Work out the finished part from the listing and answer in its coordinate system (mm). Round coordinates to 2 decimals unless told otherwise and drop trailing zeros. Write each loop counter-clockwise with the first axis right and the second up, starting at its lowest first coordinate (ties: lowest second). Pieces come first, ordered by that corner, then holes. Notation, with made-up numbers: (76, 21) - (135, 21) arc R27 cw to (135, 48) - close; hole circle Ø2 at (-19.75, 52.5). An arc over 180 degrees is marked (long way). Answer as a JSON object with one key per item and string values.
```python
from build123d import *

# Parameters (mm, degrees)
SKETCH2_W           = 200
SKETCH2_H           = 20
BOSS_EXTRUDE1_DEPTH = 3
SKETCH3_R           = 3
CUT_EXTRUDE1_DEPTH  = 202.019899512
SKETCH4_R           = 3
CUT_EXTRUDE2_DEPTH  = 202.019899512
FILLET1_R           = 10
FILLET2_R           = 10
SKETCH6_R           = 3
CUT_EXTRUDE3_DEPTH  = 202.019899512


with BuildPart() as part:
    # Sketch2 → Boss-Extrude1 (new body)
    with BuildSketch(Plane(origin=(0, 0, 0), x_dir=(1, 0, 0), z_dir=(0, 1, 0))):
        with Locations((100, 10)):
            Rectangle(SKETCH2_W, SKETCH2_H)
    extrude(amount=BOSS_EXTRUDE1_DEPTH)

    # Sketch3 → Cut-Extrude1 (cut, through all)
    with BuildSketch(Plane(origin=(0, 3, 0), x_dir=(1, 0, 0), z_dir=(0, 1, 0))):
        with Locations(Location((9, 10, 0), (0, 0, 270))):
            Circle(SKETCH3_R)
    extrude(amount=-CUT_EXTRUDE1_DEPTH, mode=Mode.SUBTRACT)

    # Sketch4 → Cut-Extrude2 (cut, through all)
    with BuildSketch(Plane(origin=(0, 3, 0), x_dir=(1, 0, 0), z_dir=(0, 1, 0))):
        with Locations(Location((191, 10, 0), (0, 0, 270))):
            Circle(SKETCH4_R)
    extrude(amount=-CUT_EXTRUDE2_DEPTH, mode=Mode.SUBTRACT)

    # Fillet1
    fillet1_edges = [part.edges().sort_by_distance(p)[0] for p in [
        (0, 1.5, -20),
        (0, 1.5, 0),
    ]]
    fillet(fillet1_edges, radius=FILLET1_R - 0.0001)  # a hair under: the kernel refuses the full size

    # Fillet2
    fillet2_edges = [part.edges().sort_by_distance(p)[0] for p in [
        (200, 1.5, -20),
        (200, 1.5, 0),
    ]]
    fillet(fillet2_edges, radius=FILLET2_R - 0.0001)  # a hair under: the kernel refuses the full size

    # Sketch6 → Cut-Extrude3 (cut, through all)
    with BuildSketch(Plane(origin=(0, 3, 0), x_dir=(1, 0, 0), z_dir=(0, 1, 0))):
        with Locations(Location((100, 10, 0), (0, 0, 270))):
            Circle(SKETCH6_R)
    extrude(amount=-CUT_EXTRUDE3_DEPTH, mode=Mode.SUBTRACT)


solid = part.part
```
Item 1: Determine the mould class of faces 1 (the cylindrical face through (196.99, 1.52, -2.85)), 2 (the cylindrical face through (97.07, 1.52, -10.65)), 3 (the flat face through (99, 3, -15)), 4 (the cylindrical face through (2.85, 1.52, -3.01)) for opening direction X: pulls with the +X half, pulls with the -X half, needs draft (parallel to the pull), parting line crosses it, or undercut.
Results found:
{"face 1": "pulls with the +X half", "face 2": "undercut", "face 3": "needs draft", "face 4": "pulls with the -X half"}
Item 2: A cutting plane is placed at A-A (x = 100). Write down the section's boundary in (y, z).
Results found:
{"outline": "(0, -20) - (3, -20) - (3, -13) - (0, -13) - close; (0, -7) - (3, -7) - (3, 0) - (0, 0) - close"}
Item 3: A cutting plane is placed at C-C (z = -2.75). Write down the section's boundary in (x, y), and give its area (3 significant figures).
Results found:
{"outline": "(3.11, 0) - (196.89, 0) - (196.89, 3) - (3.11, 3) - close", "area": "581 mm²"}
Item 4: A cutting plane is placed at B-B (y = 1.15). Give the number of separate pieces and of enclosed holes in the cut face, and give its area (3 significant figures).
Results found:
{"separate pieces": "1", "enclosed holes": "3", "area": "3,830 mm²"}
Item 5: Consider line 1 along X through (y, z) = (0.9, -10); line 2 along Z through (x, y) = (191.5, 0.95); line 3 along Z through (x, y) = (8, 0.85). Determine where each line is inside the solid, lowest interval first.
Results found:
{"line 1": "0 to 6, 12 to 97, 103 to 188, 194 to 200", "line 2": "-19.89 to -12.96, -7.04 to -0.11", "line 3": "-19.8 to -12.83, -7.17 to -0.2"}
